For this review, take the finished solid that the model builds, in its own axes (mm). A direction names the side the tool comes from. Give positions to 0.01 mm unless a question says otherwise; leave off trailing zeros. Write each loop counter-clockwise with the first axis right and the second up, starting at its lowest first coordinate (ties: lowest second). Pieces come first, ordered by that corner, then holes.
1) For P1, Ø3, axis at y = 5, z = 4.76, coming from the -X side; P2, Ø3.5, axis at x = 0, y = 0, coming from the -Z side; P3, Ø1, axis at y = -4.5, z = 4.5, coming from the +X side, all flat-tipped, find the tip position at first contact; note any pin that passes through.
2) We need section D-D on y = 6.25. Give the boundary of the cut face in (x, z) (1 decimal).
3) We need section B-B on y = 0. Give the boundary of the cut face in (x, z) (1 decimal), and give its area (3 significant figures).
4) Draft analysis for pull direction Z (two halves, no side actions). For faces 1 (the face through (-3, 0, 0)), 2 (the face through (10.482, 6.708, 4.383)), 3 (the face through (-3, 0, 9.525)), 4 (the face through (0, -9, 5)), state which applies: pulls with the +Z half, pulls with the -Z half, needs draft (parallel to the pull), parting line crosses it, or undercut.
5) We need section A-A on x = 0. Give the boundary of the cut face in (y, z) (3 decimals).
6) Machinability: for faces 5 (the face through (6.538, -5, 5)), 6 (the face through (-6.538, 5, 5)), 7 (the face through (0, 9, 5)), which of the approach directions +Z, -Z, +X, -X, +Y, -Y give a long, thin tool a straight path to every point of the face, cutting with its end or side? Answer none if there is none.
7) Wall thickness on line 1 along Z through (x, y) = (-10.25, -5) (1 decimal); line 2 along Y through (x, z) = (-9.75, 3.5); line 3 along X through (y, z) = (5.5, 5.5): over which ranges is each line inside the solid? List them lowest first.
8) We need section C-C on x = -11.5. Give the number of separate pieces and of enclosed holes in the cut face, and give its area (3 significant figures).
from build123d import *

# Parameters (mm, degrees)
SKETCH1_W         = 29.075
SKETCH1_H         = 18
EXTRUDE_3_8_DEPTH = 9.525
SKETCH2_R         = 1.75
M4_DRILL_DEPTH    = 8
M4_DRILL2_START   = -8
SKETCH3_R         = 1.75
M4_DRILL2_DEPTH   = 8
SKETCH5_R         = 2.2
M5_DRILL_DEPTH    = 9.525


with BuildPart() as part:
    # Sketch1 → 3/8 (new body)
    with BuildSketch(Plane.XY):
        Rectangle(SKETCH1_W, SKETCH1_H)
    extrude(amount=EXTRUDE_3_8_DEPTH)

    # Sketch2 → M4_DRILL (cut)
    with BuildSketch(Plane.ZY.offset(14.5375)):
        with Locations((4.7625, 5)):
            Circle(SKETCH2_R)
        with Locations(Location((4.7625, -5, 0), (0, 0, 180))):
            Circle(SKETCH2_R)
    extrude(amount=-M4_DRILL_DEPTH, mode=Mode.SUBTRACT)

    # Sketch3 → M4_DRILL2 (cut)
    with BuildSketch(Plane(origin=(14.5375, 0, 0), x_dir=(0, 0, -1), z_dir=(1, 0, 0)).offset(M4_DRILL2_START)):
        with Locations((-4.7625, -5)):
            Circle(SKETCH3_R)
        with Locations(Location((-4.7625, 5, 0), (0, 0, 180))):
            Circle(SKETCH3_R)
    extrude(amount=M4_DRILL2_DEPTH, mode=Mode.SUBTRACT)

    # Sketch5 → M5_DRILL (cut)
    with BuildSketch(Plane(origin=(0, 0, 0), x_dir=(-1, 0, 0), z_dir=(0, 0, -1))):
        Circle(SKETCH5_R)
    extrude(amount=-M5_DRILL_DEPTH, mode=Mode.SUBTRACT)


solid = part.part
Results list:
1. P1: stops at x = -6.54
1. P2: passes through
1. P3: stops at x = 6.54
2. outline: (-14.5, 0) - (14.5, 0) - (14.5, 3.5) - (6.5, 3.5) - (6.5, 6) - (14.5, 6) - (14.5, 9.5) - (-14.5, 9.5) - (-14.5, 6) - (-6.5, 6) - (-6.5, 3.5) - (-14.5, 3.5) - close
3. outline: (-14.5, 0) - (-2.2, 0) - (-2.2, 9.5) - (-14.5, 9.5) - close; (2.2, 0) - (14.5, 0) - (14.5, 9.5) - (2.2, 9.5) - close
3. area: 235 mm2
4. face 1: pulls with the -Z half
4. face 2: undercut
4. face 3: pulls with the +Z half
4. face 4: needs draft
5. outline: (-9, 0) - (-2.2, 0) - (-2.2, 9.525) - (-9, 9.525) - close; (2.2, 0) - (9, 0) - (9, 9.525) - (2.2, 9.525) - close
6. face 5: +X
6. face 6: -X
6. face 7: +Z, -Z, +X, -X, +Y
7. line 1: z = 0 to 3, 6.5 to 9.5
7. line 2: y = -9 to -6.21, -3.79 to 3.79, 6.21 to 9
7. line 3: x = -6.54 to 6.54
8. separate pieces: 1
8. enclosed holes: 2
8. area: 152 mm2
